Here's how the part is built. I have some questions about the finished solid (model axes, mm). Face numbers are marked on the shaded views. A direction names the side the tool comes from. Coordinates: 2 decimals unless noted, no trailing zeros. Write each loop counter-clockwise with the first axis right and the second up, starting at its lowest first coordinate (ties: lowest second). Pieces come first, ordered by that corner, then holes. Notation, with made-up numbers: (10.5, -4) -> (54.5, -4) arc R18 ccw to (54.5, 13) -> close; hole circle Ø8 at (9, 7). An arc over 180 degrees is marked (long way). Put each result on its own line as item: value. Start each with the question number.
Item 1: If we mould it in two halves opening along Y, with no side actions, what happens to the marked faces 1, 2, 3 and 4? For each: released by +Y, released by -Y, zero draft, split by the parting line, or undercut.
Item 2: I need wall thicknesses on line 1 (Y direction, x = 0, z = 6.25); line 2 (Z direction, x = 4, y = -10); line 3 (Y direction, x = -3, z = 4). Which ranges of each line are inside material? Lowest first, please. Write a range as [from, to].
Item 3: I want a section at A-A, the plane y = 0. List the corners of the cut face in (x, z) for me, then the cut area to 3 significant figures.
Item 4: I want a section at C-C, the plane x = -8. List the corners of the cut face in (y, z) for me, then the cut area to 3 significant figures.
Item 5: I want a section at D-D, the plane y = 5.5. List the corners of the cut face in (x, z) for me, then the cut area to 3 significant figures.
Item 6: For pin 1 (8 mm diameter, centred on x = -25, y = 0, fed in from +Z); pin 2 (4 mm diameter, centred on x = 21.5, z = 1.5, fed in from -Y); pin 3 (2 mm diameter, centred on x = -23.5, z = 6, fed in from +Y); pin 4 (2 mm diameter, centred on y = 5.5, z = 9, fed in from +X), each with a flat end and sliding along its axis, tell me the tip position at first contact or that it passes through.
Item 7: On a 3-axis mill with a long thin cutter (end or side, diameter ignored), from which of +Z, -Z, +X, -X, +Y, -Y can I reach the whole of each face in a straight line? I mean the marked faces 5 and 6. Say none if no direction works.
Item 8: I want a section at B-B, the plane z = 8.75. List the corners of the cut face in (x, y) for me.
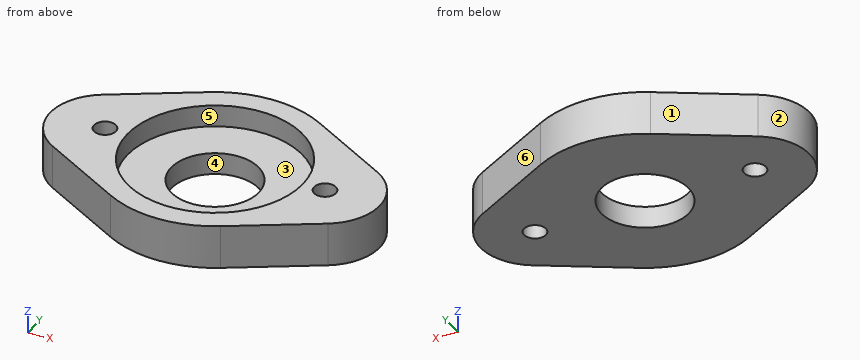
from build123d import *

# Parameters (mm, degrees)
EXTRUDE_1_DEPTH     = 10
SKETCH_2_R          = 20
CUT_EXTRUDE_1_DEPTH = 5
CUT_EXTRUDE_2_REACH = 47.346
SKETCH_3_R          = 10
CUT_EXTRUDE_3_REACH = 48.165
SKETCH_4_R          = 2.5


with BuildPart() as part:
    # 草图1 → 凸台-拉伸1 (new body)
    with BuildSketch(Plane.XY):
        with BuildLine():
            Line((12.5, 21.650635095), (31.25, 10.825317547))
            ThreePointArc((31.25, 10.825317547), (37.5, 0), (31.25, -10.825317547))
            Line((31.25, -10.825317547), (12.5, -21.650635095))
            ThreePointArc((12.5, -21.650635095), (0, -25), (-12.5, -21.650635095))
            Line((-12.5, -21.650635095), (-31.25, -10.825317547))
            ThreePointArc((-31.25, -10.825317547), (-37.5, 0), (-31.25, 10.825317547))
            Line((-31.25, 10.825317547), (-12.5, 21.650635095))
            ThreePointArc((-12.5, 21.650635095), (0, 25), (12.5, 21.650635095))
        make_face()
    extrude(amount=EXTRUDE_1_DEPTH)

    # 草图2 → 切除-拉伸1 (cut)
    with BuildSketch(Plane.XY.offset(10)):
        Circle(SKETCH_2_R)
    extrude(amount=-CUT_EXTRUDE_1_DEPTH, mode=Mode.SUBTRACT)

    # 草图3 → 切除-拉伸2 (cut, up to next)
    with BuildSketch(Plane.XY.offset(5), mode=Mode.PRIVATE) as cut_extrude_2_sk1:
        Circle(SKETCH_3_R)
    cut_extrude_2_tool1 = extrude(cut_extrude_2_sk1.sketch, amount=-CUT_EXTRUDE_2_REACH, mode=Mode.PRIVATE) & part.part
    add(cut_extrude_2_tool1.solids().sort_by_distance((0, 0, 5))[0], mode=Mode.SUBTRACT)

    # 草图4 → 切除-拉伸3 (cut, up to next)
    with BuildSketch(Plane.XY.offset(10), mode=Mode.PRIVATE) as cut_extrude_3_sk1:
        with Locations((-25, 0)):
            Circle(SKETCH_4_R)
    cut_extrude_3_tool1 = extrude(cut_extrude_3_sk1.sketch, amount=-CUT_EXTRUDE_3_REACH, mode=Mode.PRIVATE) & part.part
    cut_extrude_3 = cut_extrude_3_tool1.solids().sort_by_distance((-25, 0, 10))[0]
    add(cut_extrude_3, mode=Mode.SUBTRACT)

    # 镜向1: 切除-拉伸3 across plane
    add(cut_extrude_3.mirror(Plane(origin=(0, 0, 0), x_dir=(0, 0, 1), z_dir=(1, 0, 0))), mode=Mode.SUBTRACT)


solid = part.part
Calculated:
1. face 1: released by +Y
1. face 2: split by the parting line
1. face 3: undercut
1. face 4: undercut
2. line 1: y = [-25, -20], [20, 25]
2. line 2: z = [0, 5]
2. line 3: y = [-24.82, -9.54], [9.54, 24.82]
3. outline: (-37.5, 0) -> (-27.5, 0) -> (-27.5, 10) -> (-37.5, 10) -> close; (-22.5, 0) -> (-10, 0) -> (-10, 5) -> (-20, 5) -> (-20, 10) -> (-22.5, 10) -> close; (10, 0) -> (22.5, 0) -> (22.5, 10) -> (20, 10) -> (20, 5) -> (10, 5) -> close; (27.5, 0) -> (37.5, 0) -> (37.5, 10) -> (27.5, 10) -> close
3. area: 350 mm2
4. outline: (-23.69, 0) -> (-6, 0) -> (-6, 5) -> (-18.33, 5) -> (-18.33, 10) -> (-23.69, 10) -> close; (6, 0) -> (23.69, 0) -> (23.69, 10) -> (18.33, 10) -> (18.33, 5) -> (6, 5) -> close
4. area: 230 mm2
5. outline: (-36.22, 0) -> (-8.35, 0) -> (-8.35, 5) -> (-19.23, 5) -> (-19.23, 10) -> (-36.22, 10) -> close; (8.35, 0) -> (36.22, 0) -> (36.22, 10) -> (19.23, 10) -> (19.23, 5) -> (8.35, 5) -> close
5. area: 449 mm2
6. pin 1: stops at z = 10
6. pin 2: stops at y = -17.61
6. pin 3: stops at y = 15.88
6. pin 4: stops at x = 36.66
7. face 5: +Z
7. face 6: +Z, -Z, +X, +Y
8. outline: (-31.25, -10.83) -> (-12.5, -21.65) arc R25 ccw to (12.5, -21.65) -> (31.25, -10.83) arc R12.5 ccw to (31.25, 10.83) -> (12.5, 21.65) arc R25 ccw to (-12.5, 21.65) -> (-31.25, 10.83) arc R12.5 ccw to start; hole circle Ø5 at (-25, 0); hole circle Ø40 at (0, 0); hole circle Ø5 at (25, 0)
